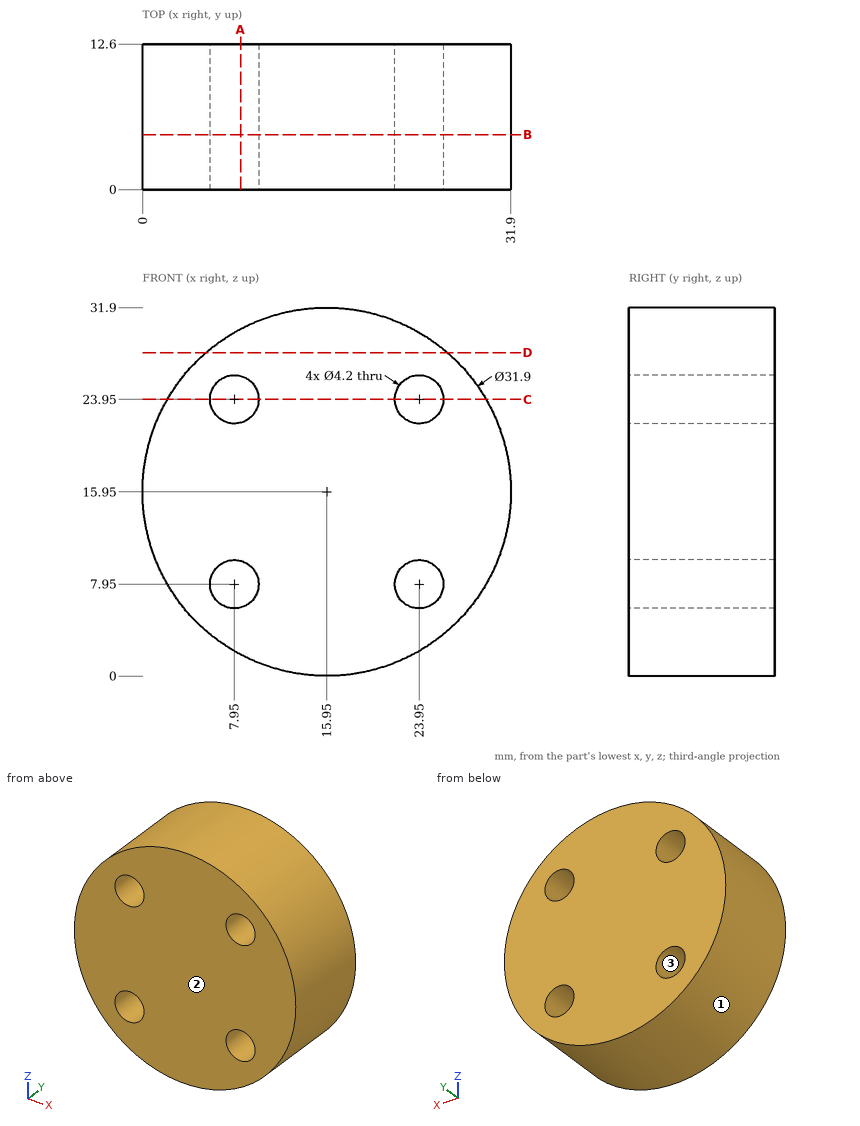
The drawing under review shows one solid part. Ordinate dimensions are in mm from its lowest x, y, z. Round coordinates to 2 decimals unless told otherwise and drop trailing zeros. Loops run counter-clockwise (first coordinate to the right, second up) from the corner with the lowest first, then second, coordinate; pieces in that order, holes last. Notation, with made-up numbers: (47, -36.5) - (73, -36.5) arc R29 cw to (73, 2.5) - close; hole circle Ø1 at (-1.75, 4). An arc over 180 degrees is marked (long way). Put each result on its own line as item: value. Start each with the question number.
1. Insertion check: P1, Ø1, axis at x = 14, y = 7, coming from the +Z side; P2, Ø5, axis at y = 3, z = 25.5, coming from the +X side; P3, Ø5.5, axis at x = 7.95, z = 7.95, coming from the +Y side; P4, Ø5, axis at x = 27.5, y = 11, coming from the -Z side. Each pin has a flat end and moves straight along its axis. Give the tip position at first contact, or say it passes through.
2. Consider section C-C on z = 23.95. State the section outline as (x, y) points.
3. Consider section D-D on z = 28. State the section outline as (x, y) points.
4. Consider section B-B on y = 4.75. State the section outline as (x, z) points, plus the area to 3 significant figures.
5. Consider section A-A on x = 8.5. State the section outline as (y, z) points, plus the area to 3 significant figures.
6. Mouldability with a two-part tool opening along Z and no side actions: class the marked faces 1, 2 and 3 as +Z half, -Z half, draft (parallel to the pull), parting line (faces both ways), or undercut.
7. For probe 1 along Z at (x, y) = (23.95, 5.5); probe 2 along X at (y, z) = (9.5, 23); probe 3 along X at (y, z) = (3.5, 7), list the stretches that pass through material, from the lowest coordinate up. Write a range as [from, to].
Result sheet:
1. P1: z = 31.83
1. P2: x = 30.26
1. P3: y = 12.6
1. P4: z = 2.82
2. outline: (2.15, 0) - (5.85, 0) - (5.85, 12.6) - (2.15, 12.6) - close; (10.05, 0) - (21.85, 0) - (21.85, 12.6) - (10.05, 12.6) - close; (26.05, 0) - (29.75, 0) - (29.75, 12.6) - (26.05, 12.6) - close
3. outline: (5.5, 0) - (26.4, 0) - (26.4, 12.6) - (5.5, 12.6) - close
4. outline: circle Ø31.9 at (15.95, 15.95); hole circle Ø4.2 at (7.95, 7.95); hole circle Ø4.2 at (7.95, 23.95); hole circle Ø4.2 at (23.95, 7.95); hole circle Ø4.2 at (23.95, 23.95)
4. area: 744 mm^2
5. outline: (0, 1.85) - (12.6, 1.85) - (12.6, 5.92) - (0, 5.92) - close; (0, 9.98) - (12.6, 9.98) - (12.6, 21.92) - (0, 21.92) - close; (0, 25.98) - (12.6, 25.98) - (12.6, 30.05) - (0, 30.05) - close
5. area: 253 mm^2
6. face 1: parting line
6. face 2: draft
6. face 3: undercut
7. probe 1: [2.15, 5.85], [10.05, 21.85], [26.05, 29.75]
7. probe 2: [1.64, 6.08], [9.82, 22.08], [25.82, 30.26]
7. probe 3: [2.75, 6.08], [9.82, 22.08], [25.82, 29.15]
